Geometry check sheet. Reference: the model listing, model coordinates, mm. Coordinates: 2 decimals unless noted, no trailing zeros. Write each loop counter-clockwise with the first axis right and the second up, starting at its lowest first coordinate (ties: lowest second). Pieces come first, ordered by that corner, then holes.
from build123d import *

# Parameters (mm, degrees)
SKETCH_1_W          = 30
SKETCH_1_H          = 30
EXTRUDE_1_DEPTH     = 36
CUT_EXTRUDE_START   = -15.811192309
CUT_EXTRUDE_9_DEPTH = 30


# Read off the part's stored shape, not the designer's step: 切除-拉伸9
with BuildPart() as part:
    # 草图1 → 凸台-拉伸1 (new body)
    with BuildSketch(Plane(origin=(0, 0, 0), x_dir=(1, 0, 0), z_dir=(0, 1, 0))):
        with Locations((0.922994888, 0.811192309)):
            Rectangle(SKETCH_1_W, SKETCH_1_H)
    extrude(amount=EXTRUDE_1_DEPTH)

    # 切除-拉伸9 outline → 切除-拉伸9 (cut)
    with BuildSketch(Plane.XY.offset(CUT_EXTRUDE_START)):
        Polygon((-14.077005112, 36), (-14.077005112, 21.665729015), (0.922994888, 36), align=None)
        Polygon((15.922994888, 36), (0.922994888, 36), (15.922994888, 21.379503866), align=None)
    extrude(amount=CUT_EXTRUDE_9_DEPTH, mode=Mode.SUBTRACT)


solid = part.part
1. Draft check along Z on faces 1 (the flat face through (8.32, 28.79, -1.02)), 2 (the flat face through (1, 14, -15.811)), 3 (the flat face through (1, 14, 14.189)). Enter one of: released by +Z, released by -Z, zero draft, split by the parting line, or undercut.
Computed values:
face 1: zero draft
face 2: released by -Z
face 3: released by +Z
2. Sectioned sample at A-A, the plane z = -3.75. Record the boundary of the cut face in (x, y).
Computed values:
outline: (-14.08, 0) - (15.92, 0) - (15.92, 21.38) - (0.92, 36) - (-14.08, 21.67) - close
3. Gauge pin test, flat ends, axial feed: pin 1 Ø3 at (y, z) = (25.5, 6.5) entering from +X; pin 2 Ø6 at (y, z) = (31, -5.5) entering from +X; pin 3 Ø12 at (y, z) = (31, -9.5) entering from -X. Record the tip position at first contact, or that the pin passes through.
Computed values:
pin 1: stops at x = 13.23
pin 2: stops at x = 9.13
pin 3: stops at x = -10.59
4. Thickness scan on line 1 along Y through (x, z) = (3.25, -9.5); line 2 along Y through (x, z) = (11.5, -2.25); line 3 along X through (y, z) = (28.5, 2.75). Record the ranges inside material, lowest first.
Computed values:
line 1: y = 0 to 33.73
line 2: y = 0 to 25.69
line 3: x = -6.93 to 8.62
5. Sectioned sample at C-C, the plane x = -4. Record the boundary of the cut face in (y, z).
Computed values:
outline: (0, -15.81) - (31.3, -15.81) - (31.3, 14.19) - (0, 14.19) - close
6. Sectioned sample at B-B, the plane y = 22.5. Record the boundary of the cut face in (x, z), and give its area (3 significant figures).
Computed values:
outline: (-13.2, -15.81) - (14.77, -15.81) - (14.77, 14.19) - (-13.2, 14.19) - close
area: 839 mm2
